Source: CAD feature listing. Evaluate the final solid. Frame: model axes, mm. A direction names the side the tool comes from. Give positions to 0.01 mm unless a question says otherwise; leave off trailing zeros. Order: outer loops, then holes, each group sorted by start corner. A loop starts at its lowest first (then second) coordinate and runs counter-clockwise, first axis right, second up.
```python
from build123d import *

# Parameters (mm, degrees)
SKETCH2_W               = 74.64
SKETCH2_H               = 49.9
SKETCH2_R               = 11.05
BOSS_EXTRUDE3_DEPTH     = 49.22
BOSS_EXTRUDE4_DEPTH     = 49.22
SKETCH7_R               = 5.95
BOSS_EXTRUDE5_DEPTH     = 12.67
SKETCH8_R               = 3.35
BOSS_EXTRUDE6_DEPTH     = 10.6
SKETCH9_R               = 2.447157839
CUT_EXTRUDE1_DEPTH      = 4
CUT_EXTRUDE2_DEPTH      = 145.004745584
CUT_EXTRUDE2_DEPTH_BACK = 4
SKETCH11_R              = 3.585
CUT_EXTRUDE3_DEPTH      = 2
SKETCH12_R              = 3.585
CUT_EXTRUDE4_DEPTH      = 2
SKETCH13_R              = 3.585
CUT_EXTRUDE5_DEPTH      = 2


with BuildPart() as part:
    # Sketch2 → Boss-Extrude3 (new body)
    with BuildSketch(Plane.XY):
        with Locations((-36.171052169, 23.819106833)):
            Rectangle(SKETCH2_W, SKETCH2_H)
        with Locations((-56.191052169, 31.609453319)):
            Circle(SKETCH2_R, mode=Mode.SUBTRACT)
    extrude(amount=BOSS_EXTRUDE3_DEPTH)

    # Sketch3 → Boss-Extrude4 (add)
    with BuildSketch(Plane.XY):
        with BuildLine():
            Line((-73.491052169, 48.769106833), (-113.415991852, 25.422550529))
            add(Edge.make_bspline(
                [(-73.491052169, -1.130893167), (-103.22071341, -0.46361186), (-113.415991852, 25.422550529)],
                knots=[0, 0, 0, 1, 1, 1], degree=2))
            Line((-73.491052169, -1.130893167), (-73.491052169, 48.769106833))
        make_face()
    extrude(amount=BOSS_EXTRUDE4_DEPTH)

    # Sketch7 → Boss-Extrude5 (add)
    with BuildSketch(Plane(origin=(0, 48.769106833, 0), x_dir=(1, 0, 0), z_dir=(0, 1, 0))):
        with Locations(Location((-23.531052169, -22.62, 0), (0, 0, 90))):
            Circle(SKETCH7_R)
    extrude(amount=BOSS_EXTRUDE5_DEPTH)

    # Sketch8 → Boss-Extrude6 (add)
    with BuildSketch(Plane(origin=(0, 61.439106833, 0), x_dir=(1, 0, 0), z_dir=(0, 1, 0))):
        with Locations(Location((-23.531052169, -22.62, 0), (0, 0, 270))):
            Circle(SKETCH8_R)
    extrude(amount=BOSS_EXTRUDE6_DEPTH)

    # Sketch9 → Cut-Extrude1 (cut)
    with BuildSketch(Plane(origin=(0, 72.039106833, 0), x_dir=(1, 0, 0), z_dir=(0, 1, 0))):
        with Locations(Location((-23.531052169, -22.62, 0), (0, 0, 270))):
            Circle(SKETCH9_R)
    extrude(amount=-CUT_EXTRUDE1_DEPTH, mode=Mode.SUBTRACT)

    # Sketch10 → Cut-Extrude2 (cut, two sides: drawn at the far end of the back side and taken through both)
    with BuildSketch(Plane(origin=(1.148947831, 0, 0), x_dir=(0, 0, -1), z_dir=(1, 0, 0)).offset(-CUT_EXTRUDE2_DEPTH_BACK)):
        Polygon((-33.176264777, 183.063086359), (-33.176264777, 48.769106833), (-33.176264777, 32.869106833), (-12.176264777, 32.869106833), (-12.176264777, 48.769106833), (-12.176264777, 183.063086359), (-12.176264777, 451.651045412), (-33.176264777, 451.651045412), align=None)
    extrude(amount=CUT_EXTRUDE2_DEPTH + CUT_EXTRUDE2_DEPTH_BACK, mode=Mode.SUBTRACT)

    # Sketch11 → Cut-Extrude3 (cut)
    with BuildSketch(Plane(origin=(-2.851052169, 0, 0), x_dir=(0, 0, -1), z_dir=(1, 0, 0))):
        with Locations(Location((-22.624143427, 40.627842238, 0), (0, 0, 90))):
            Circle(SKETCH11_R)
    extrude(amount=-CUT_EXTRUDE3_DEPTH, mode=Mode.SUBTRACT)

    # Sketch12 → Cut-Extrude4 (cut)
    with BuildSketch(Plane(origin=(1.148947831, 0, 0), x_dir=(0, 0, -1), z_dir=(1, 0, 0))):
        with Locations(Location((-9.6, 28.719106833, 0), (0, 0, 90))):
            Circle(SKETCH12_R)
    extrude(amount=-CUT_EXTRUDE4_DEPTH, mode=Mode.SUBTRACT)

    # Sketch13 → Cut-Extrude5 (cut)
    with BuildSketch(Plane(origin=(1.148947831, 0, 0), x_dir=(0, 0, -1), z_dir=(1, 0, 0))):
        with Locations(Location((-37.02, 28.719106833, 0), (0, 0, 90))):
            Circle(SKETCH13_R)
    extrude(amount=-CUT_EXTRUDE5_DEPTH, mode=Mode.SUBTRACT)


solid = part.part
```
1) Draft query along Y for faces 5 (the flat face through (-93.17, 37.26, 24.27)), 6 (the flat face through (-2.851, 44.5, 22.8)), 7 (the cylindrical face through (0.163, 30.373, 6.419)). Return one class per face: +Y half, -Y half, draft (parallel to the pull), parting line (faces both ways), or undercut.
Report:
face 5: +Y half
face 6: draft
face 7: undercut
2) Section query B-B, the plane y = 57. Return the cut outline in (x, z), and give its area (3 significant figures).
Report:
outline: circle Ø11.9 at (-23.53, 22.62)
area: 111 mm2
3) Reachability of faces 1 (the cylindrical face through (-24.814, 66.665, 25.715)), 2 (the flat face through (-1, 41, 12.176)), 3 (the flat face through (-44, 24, 0)), 4 (the flat face through (-4.851, 41, 23)) from +Z, -Z, +X, -X, +Y, -Y: full face, straight path, thin tool, end or side. Return the list, or none.
Report:
face 1: +Y
face 2: +X, +Y
face 3: -Z, +X, -X, +Y, -Y
face 4: +X
4) Section query A-A, the plane x = -71. Return the cut outline in (y, z), and give its area (3 significant figures).
Report:
outline: (-1.13, 0) - (48.77, 0) - (48.77, 49.22) - (-1.13, 49.22) - close
area: 2,460 mm2
5) Material intervals for L1, parallel to Y at x = 0, z = 37; L2, parallel to Y at x = -14, z = 43; L3, parallel to Y at x = 0, z = 9, sorted ascending.
Report:
L1: y = -1.13 to 25.13, 32.3 to 48.77
L2: y = -1.13 to 48.77
L3: y = -1.13 to 25.18, 32.25 to 48.77
6) Pin query (flat end, axial travel): pin 1 (1.5 mm diameter, centred on x = -23.5, z = 23, fed in from +Y); pin 2 (4.5 mm diameter, centred on y = 28.72, z = 9.6, fed in from -X); pin 3 (5.5 mm diameter, centred on y = 40.63, z = 22.62, fed in from +X). Return the tip coordinate at first contact, or that it passes through.
Report:
pin 1: stops at y = 68.04
pin 2: stops at x = -111.62
pin 3: stops at x = -4.85
